from build123d import *

# Parameters (mm, degrees)
SKETCH_1_R      = 0.6
EXTRUDE_1_DEPTH = 15
SKETCH_2_R      = 0.60381225
SKETCH_2_R_2    = 0.602112423
EXTRUDE_2_DEPTH = 2.5


with BuildPart() as part:
    # 草图1 → 凸台-拉伸1 (new body)
    with BuildSketch(Plane(origin=(0, 0, 0), x_dir=(0, 0, -1), z_dir=(1, 0, 0))):
        Circle(SKETCH_1_R)
    extrude(amount=EXTRUDE_1_DEPTH)

    # 草图2 → 凸台-拉伸2 (add, symmetric)
    with BuildSketch(Plane.XY):
        with Locations((15.00822403, 0)):
            Circle(SKETCH_2_R)
        Circle(SKETCH_2_R_2)
    extrude(amount=EXTRUDE_2_DEPTH, both=True)


solid = part.part
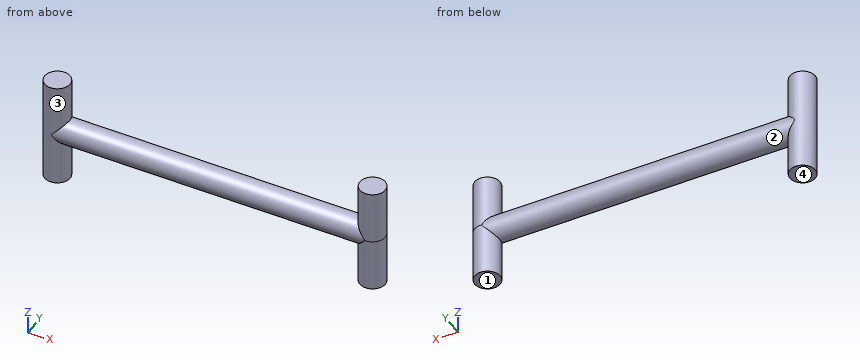
The listing builds one solid part. Answer for the finished solid, in the listing's coordinates (mm). Face numbers are marked on the shaded views. A direction names the side the tool comes from. Give positions to 0.01 mm unless a question says otherwise; leave off trailing zeros. Write each loop counter-clockwise with the first axis right and the second up, starting at its lowest first coordinate (ties: lowest second). Pieces come first, ordered by that corner, then holes. Notation, with made-up numbers: (75.25, -23) - (131.25, -23) arc R19 ccw to (131.25, 14) - close; hole circle Ø2 at (41, 24.25). An arc over 180 degrees is marked (long way). One line per question, with ' | ' between items. Start each with the question number.
1. Section C-C, the plane x = 6.25 is taken. Determine the outline of the cut face in (y, z).
2. Given P1, Ø1, axis at x = 8, z = 1.5, coming from the -Y side; P2, Ø1, axis at x = 9, z = 0.5, coming from the +Y side, each flat-ended and moving along its own axis, determine where each tip first touches the part or whether it passes through.
3. Section B-B, the plane z = -1.8 is taken. Determine the outline of the cut face in (x, y).
4. Straight lines are drawn through the part: line 1 (X direction, y = 0.05, z = -1.3); line 2 (X direction, y = 0.4, z = -0.75); line 3 (Y direction, x = 4.25, z = 0.15). For each, find the intervals that lie inside material, in ascending order.
5. For the marked faces 3 and 4, determine the directions among +Z, -Z, +X, -X, +Y, -Y from which every point of the face is accessible in a straight line to the end or side of a thin tool.
6. Section A-A, the plane y = 0.25 is taken. Determine the outline of the cut face in (x, z).
7. Section D-D, the plane y = -0.35 is taken. Determine the outline of the cut face in (x, z).
8. Determine the mould class of the marked faces 1 and 2 for opening direction X: +X half, -X half, draft (parallel to the pull), parting line (faces both ways), or undercut.
Result:
1) outline: circle Ø1.2 at (0, 0)
2) P1: passes through | P2: stops at y = 0.6
3) outline: circle Ø1.2 at (0, 0); circle Ø1.21 at (15.01, 0)
4) line 1: x = -0.6 to 0.6, 14.41 to 15.61 | line 2: x = -0.45 to 0.45, 14.56 to 15.46 | line 3: y = -0.58 to 0.58
5) face 3: none | face 4: -Z, +X, -X, +Y, -Y
6) outline: (-0.55, -2.5) - (0.55, -2.5) - (0.55, -0.55) - (14.46, -0.55) - (14.46, -2.5) - (15.56, -2.5) - (15.56, 2.5) - (14.46, 2.5) - (14.46, 0.55) - (0.55, 0.55) - (0.55, 2.5) - (-0.55, 2.5) - close
7) outline: (-0.49, -2.5) - (0.49, -2.5) - (0.49, -0.49) - (14.52, -0.49) - (14.52, -2.5) - (15.5, -2.5) - (15.5, 2.5) - (14.52, 2.5) - (14.52, 0.49) - (0.49, 0.49) - (0.49, 2.5) - (-0.49, 2.5) - close
8) face 1: draft | face 2: undercut
